from build123d import *

# Parameters (mm, degrees)
SKETCH_1_R          = 2.15
EXTRUDE_1_DEPTH     = 1
EXTRUDE_2_DEPTH     = 12
SKETCH_8_R          = 1
EXTRUDE_4_DEPTH     = 2
CUT_EXTRUDE_1_DEPTH = 9
CUT_EXTRUDE_2_DEPTH = 20
SKETCH_12_R         = 3
CUT_EXTRUDE_3_DEPTH = 1
FILLET_1_R          = 20
SKETCH_13_W         = 60
SKETCH_13_H         = 50
CUT_EXTRUDE_4_DEPTH = 1


with BuildPart() as part:
    # 草图1 → 凸台-拉伸1 (new body)
    with BuildSketch(Plane(origin=(0, 0, 0), x_dir=(1, 0, 0), z_dir=(0, 1, 0))):
        with BuildLine():
            Line((-24, -22.5), (24, -22.5))
            ThreePointArc((24, -22.5), (26.828427125, -21.328427125), (28, -18.5))
            Line((28, -18.5), (28, 18.5))
            ThreePointArc((28, 18.5), (26.828427125, 21.328427125), (24, 22.5))
            Line((24, 22.5), (-24, 22.5))
            ThreePointArc((-24, 22.5), (-26.828427125, 21.328427125), (-28, 18.5))
            Line((-28, 18.5), (-28, -18.5))
            ThreePointArc((-28, -18.5), (-26.828427125, -21.328427125), (-24, -22.5))
        make_face()
        with Locations(Location((-23, 17.5, 0), (0, 0, 270))):
            Circle(SKETCH_1_R, mode=Mode.SUBTRACT)
        with Locations(Location((-23, -17.5, 0), (0, 0, 270))):
            Circle(SKETCH_1_R, mode=Mode.SUBTRACT)
        with Locations(Location((23, -17.5, 0), (0, 0, 270))):
            Circle(SKETCH_1_R, mode=Mode.SUBTRACT)
        with Locations(Location((23, 17.5, 0), (0, 0, 270))):
            Circle(SKETCH_1_R, mode=Mode.SUBTRACT)
    extrude(amount=EXTRUDE_1_DEPTH)

    # 草图3 → 凸台-拉伸2 (add)
    with BuildSketch(Plane(origin=(0, 1, 0), x_dir=(1, 0, 0), z_dir=(0, 1, 0))):
        with BuildLine():
            Line((-26, -13), (-26, 13))
            Line((-26, 13), (0, 13))
            ThreePointArc((0, 13), (13, 0), (0, -13))
            Line((0, -13), (-26, -13))
        make_face()
    extrude(amount=EXTRUDE_2_DEPTH)

    # 草图8 → 凸台-拉伸4 (add)
    with BuildSketch(Plane.XY.offset(13)):
        with BuildLine():
            Line((-26, 13), (-26, 40))
            ThreePointArc((-26, 40), (-22.271726092, 44.835567469), (-16.646914902, 42.459806928))
            Line((-16.646914902, 42.459806928), (0, 13))
            Line((0, 13), (-26, 13))
        make_face()
        with Locations((-21, 40)):
            Circle(SKETCH_8_R, mode=Mode.SUBTRACT)
    extrude_4 = extrude(amount=-EXTRUDE_4_DEPTH)

    # 镜向1: 凸台-拉伸4 across plane
    add(extrude_4.mirror(Plane.XY))

    # 草图9 → 切除-拉伸1 (cut)
    with BuildSketch(Plane(origin=(0, 13, 0), x_dir=(1, 0, 0), z_dir=(0, 1, 0))):
        with BuildLine():
            Line((-26, 11), (-26, -11))
            Line((-26, -11), (0, -11))
            ThreePointArc((0, -11), (11, 0), (0, 11))
            Line((0, 11), (-26, 11))
        make_face()
    extrude(amount=-CUT_EXTRUDE_1_DEPTH, mode=Mode.SUBTRACT)

    # 草图11 → 切除-拉伸2 (cut, symmetric)
    with BuildSketch(Plane.XY):
        with BuildLine():
            Line((0, 13), (13, 13))
            Line((13, 13), (13, 7))
            ThreePointArc((13, 7), (7.628297221, 8.43537945), (2.507532378, 10.601775609))
            ThreePointArc((2.507532378, 10.601775609), (1.076623467, 11.615671145), (0, 13))
        make_face()
    extrude(amount=CUT_EXTRUDE_2_DEPTH, both=True, mode=Mode.SUBTRACT)

    # 草图12 → 切除-拉伸3 (cut)
    with BuildSketch(Plane(origin=(0, 1, 0), x_dir=(1, 0, 0), z_dir=(0, 1, 0))):
        with BuildLine():
            Line((-26, -13), (0, -13))
            ThreePointArc((0, -13), (13, 0), (0, 13))
            Line((0, 13), (-26, 13))
            Line((-26, 13), (-26, -13))
        make_face()
        with Locations(Location((0, 0, 0), (0, 0, 270))):
            Circle(SKETCH_12_R, mode=Mode.SUBTRACT)
    extrude(amount=CUT_EXTRUDE_3_DEPTH, mode=Mode.SUBTRACT)

    # 圆角1
    # the kernel refuses this fillet: 20 mm, written as the material it takes off along each edge
    with BuildSketch(Plane(origin=(-26, 2, -63), x_dir=(1, 0, 0), z_dir=(0, 0, 1))) as fillet_1_piece_1:
        with BuildLine():
            CenterArc((FILLET_1_R, FILLET_1_R), FILLET_1_R, 180, 90)
            Line((0, FILLET_1_R), (0, 0))
            Line((0, 0), (FILLET_1_R, 0))
        make_face()
    extrude(amount=126, mode=Mode.SUBTRACT)

    # 草图13 → 切除-拉伸4 (cut)
    with BuildSketch(Plane.XZ):
        Rectangle(SKETCH_13_W, SKETCH_13_H)
    extrude(amount=-CUT_EXTRUDE_4_DEPTH, mode=Mode.SUBTRACT)


solid = part.part
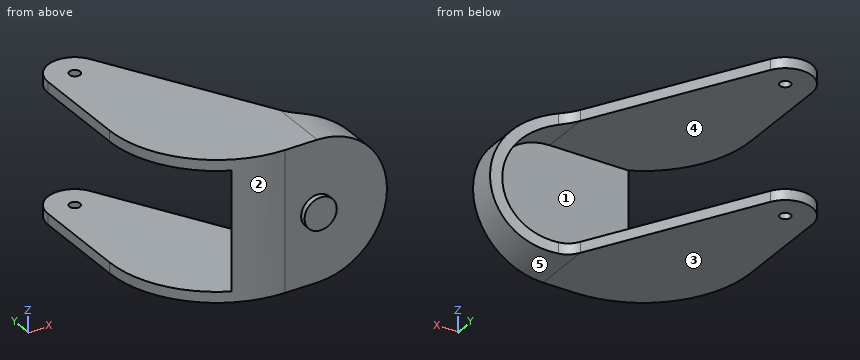
For this review, take the finished solid that the model builds, in its own axes (mm). Face numbers are marked on the shaded views. A direction names the side the tool comes from. Give positions to 0.01 mm unless a question says otherwise; leave off trailing zeros. Loops run counter-clockwise (first coordinate to the right, second up) from the corner with the lowest first, then second, coordinate; pieces in that order, holes last. Notation, with made-up numbers: M -31.75,38 L -1.75,38 A25 ccw -1.75,61 Z; hole C -2,65 d9. An arc over 180 degrees is marked long. Answer as a JSON object with one key per item and string values. Group by question number.
Q1. Tool access review of the marked faces 1 and 2: name each direction out of +Z, -Z, +X, -X, +Y, -Y from which nothing blocks a thin tool from reaching the whole face with its end or side.
Q2. Insertion check: P1, Ø4, axis at y = 6.5, z = 6, coming from the +X side; P2, Ø1, axis at x = -1.5, z = -5.5, coming from the +Y side; P3, Ø10, axis at y = 10, z = 7.5, coming from the -X side. Each pin has a flat end and moves straight along its axis. Give the tip position at first contact, or say it passes through.
Q3. Add section D-D on y = 30. Give the boundary of the cut face in (x, z).
Q4. Add section B-B on x = -21. Give the boundary of the cut face in (y, z).
Q5. Mouldability with a two-part tool opening along Z and no side actions: class the marked faces 3, 4 and 5 as +Z half, -Z half, draft (parallel to the pull), parting line (faces both ways), or undercut.
Q6. Add section A-A on y = 8. Give the boundary of the cut face in (x, z).
Q7. For probe 1 along Z at (x, y) = (-8, 23); probe 2 along Y at (x, z) = (3, -8.75); probe 3 along Y at (x, z) = (0.5, 1.5), list the stretches that pass through material, from the lowest coordinate up. Write a range as [from, to].
Q8. Add section C-C on z = 1.5. Give the boundary of the cut face in (x, y), and give its area (3 significant figures).
Checked values:
{
 "1": {"face 1": "-X, +Y", "face 2": "+Z, -Z, -X, -Y"},
 "2": {"P1": "x = 12.37", "P2": "y = 4", "P3": "x = -24.14"},
 "3": {"outline": "M -26,-13 L -9.61,-13 L -9.61,-11 L -26,-11 Z; M -26,11 L -9.61,11 L -9.61,13 L -26,13 Z"},
 "4": {"outline": "M 8.77,-13 L 39,-13 L 39,-11 L 8.77,-11 Z; M 8.77,11 L 39,11 L 39,13 L 8.77,13 Z; M 41,-13 L 45,-13 L 45,-11 L 41,-11 Z; M 41,11 L 45,11 L 45,13 L 41,13 Z"},
 "5": {"face 3": "-Z half", "face 4": "undercut", "face 5": "parting line"},
 "6": {"outline": "M -20.28,-13 L 0,-13 A13 ccw 8.97,-9.41 L 8.97,-6.36 A11 cw 0,-11 L -20.28,-11 Z; M -20.28,11 L 0,11 A11 cw 8.97,6.36 L 8.97,9.41 A13 ccw 0,13 L -20.28,13 Z"},
 "7": {"probe 1": "[-13, -11], [11, 13]", "probe 2": "[2, 4]", "probe 3": "[1, 4]"},
 "8": {"outline": "M -14.72,4 A20 ccw -6,2 L -2.6,2 L -2.6,1 L 2.6,1 L 2.6,2 L 12.91,2 L 12.91,7.02 A40 cw 10.9,7.47 L 10.9,4 Z", "area": "61.3 mm²"}
}
